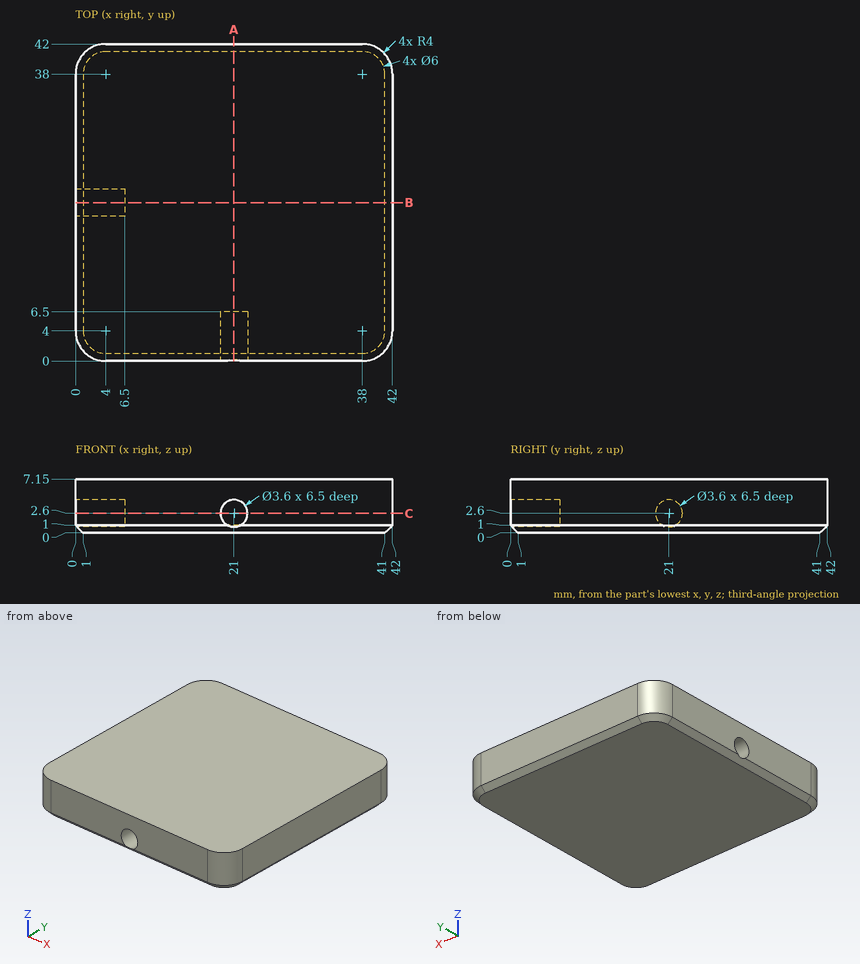
Could you check a few things on this drawing? It's one solid part, dimensions in mm from its lowest x, y, z. Coordinates: 2 decimals unless noted, no trailing zeros. Order: outer loops, then holes, each group sorted by start corner. A loop starts at its lowest first (then second) coordinate and runs counter-clockwise, first axis right, second up. Notation, with made-up numbers: (-9, -27.5) -> (12, -27.5) arc R25 cw to (12, 8.5) -> close; hole circle Ø2 at (73, 32.25). An arc over 180 degrees is marked (long way). One line per item, written item: value. Start each with the question number.
1) Imagine slicing it at A-A on x = 21. List the corners of the cut face in (y, z) for me, plus the area to 3 significant figures.
2) If I drill on L1, parallel to Z at x = 5.25, y = 21; L2, parallel to Y at x = 4.25, z = 2.6; L3, parallel to X at y = 4.5, z = 2.75, over which ranges is the centre line in solid material (lowest first)? Write a range as [from, to].
3) I'm going to push flat-ended pins straight in: pin 1 (4 mm diameter, centred on x = 21, z = 2, fed in from -Y); pin 2 (3 mm diameter, centred on x = 21, z = 2.6, fed in from -Y). Where does each tip first touch, or does it pass through?
4) Imagine slicing it at C-C on z = 2.6. List the corners of the cut face in (x, y) for me.
Answer list:
1. outline: (0, 4.4) -> (6.5, 4.4) -> (6.5, 0.8) -> (0.2, 0.8) -> (1, 0) -> (41, 0) -> (42, 1) -> (42, 7.15) -> (0, 7.15) -> close
1. area: 276 mm2
2. L1: z = [0, 0.8], [4.4, 7.15]
2. L2: y = [0, 19.2], [22.8, 42]
2. L3: x = [0, 19.21], [22.79, 42]
3. pin 1: stops at y = 0
3. pin 2: stops at y = 6.5
4. outline: (0, 4) arc R4 ccw to (4, 0) -> (19.2, 0) -> (19.2, 6.5) -> (22.8, 6.5) -> (22.8, 0) -> (38, 0) arc R4 ccw to (42, 4) -> (42, 38) arc R4 ccw to (38, 42) -> (4, 42) arc R4 ccw to (0, 38) -> (0, 22.8) -> (6.5, 22.8) -> (6.5, 19.2) -> (0, 19.2) -> close
